Input: part model. Units: mm. Frame: model coordinates. Face numbers are marked on the shaded views. A direction names the side the tool comes from. Coordinates: 2 decimals unless noted, no trailing zeros. Write each loop counter-clockwise with the first axis right and the second up, starting at its lowest first coordinate (ties: lowest second). Pieces come first, ordered by that corner, then holes.
1) Pin query (flat end, axial travel): pin 1 Ø4.5 at (y, z) = (-0.5, 18.5) entering from +X. Return the tip coordinate at first contact, or that it passes through.
2) Section query B-B (y = 0). Output: boundary loops of the cut face in (x, z), then the cut area to 3 significant figures.
3) Section query A-A (x = 11). Output: boundary loops of the cut face in (y, z).
4) Draft query along X for the marked faces 1, 2, 3 and 4. Return one class per face: pulls with the +X half, pulls with the -X half, needs draft (parallel to the pull), parting line crosses it, or undercut.
5) Set-up query: the marked faces 5, 6 and 7. Return all of +Z, -Z, +X, -X, +Y, -Y with unobstructed straight access to the full face (end or side cutting, diameter ignored); none if empty.
6) Line query: L1, parallel to Y at x = -0.5, z = 6.5; L2, parallel to X at y = 2, z = 4.75; L3, parallel to Y at x = 18, z = 14. Output: solid intervals per line, ascending.
7) Section query D-D (z = 8.5). Output: boundary loops of the cut face in (x, y).
8) Section query C-C (z = 18.75). Output: boundary loops of the cut face in (x, y).
from build123d import *

# Parameters (mm, degrees)
F0_W     = 46
F0_H     = 35
F1_DEPTH = 30
F3_DEPTH = 6.251
F4_R     = 5


with BuildPart() as f1:
    # F0 (on Top) → F1 (new body)
    with BuildSketch(Plane.XY):
        Rectangle(F0_W, F0_H)
        Polygon((-17, 7.5), (-13, 11.5), (13, 11.5), (17, 7.5), (17, -7.5), (13, -11.5), (-13, -11.5), (-17, -7.5), align=None, mode=Mode.SUBTRACT)
    extrude(amount=F1_DEPTH)

    # F2 (on face) → F3 (cut, through all)
    with BuildSketch(Plane.YZ.offset(23)):
        with BuildLine():
            Line((-7.75, 30), (-7.75, 13.75))
            ThreePointArc((-7.75, 13.75), (0, 6), (7.75, 13.75))
            Line((7.75, 13.75), (7.75, 30))
            Line((7.75, 30), (-7.75, 30))
        make_face()
    extrude(amount=-F3_DEPTH, mode=Mode.SUBTRACT)

    # F4
    f4_edges = [f1.edges().sort_by_distance(p)[0] for p in [
        (23, -17.5, 15),
        (23, 17.5, 15),
        (-23, 17.5, 15),
        (-23, -17.5, 15),
    ]]
    fillet(f4_edges, radius=F4_R)


solid = f1.part
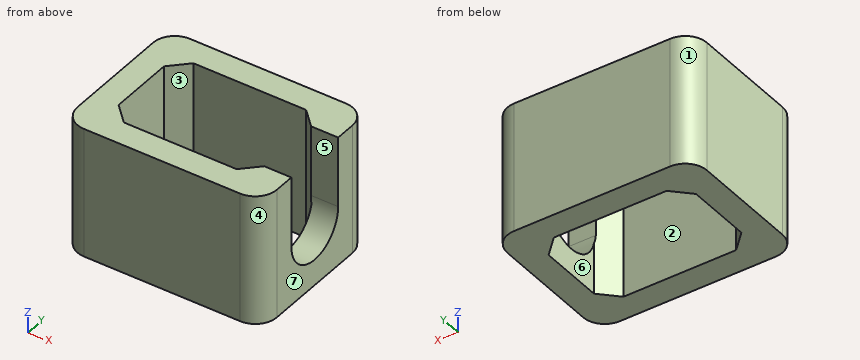
Answer:
1. pin 1: stops at x = -17
2. outline: (-23, 0) - (-17, 0) - (-17, 30) - (-23, 30) - close; (17, 0) - (23, 0) - (23, 6) - (17, 6) - close
2. area: 216 mm2
3. outline: (-17.5, 0) - (-11.5, 0) - (-11.5, 30) - (-17.5, 30) - close; (11.5, 0) - (17.5, 0) - (17.5, 30) - (11.5, 30) - close
4. face 1: pulls with the -X half
4. face 2: undercut
4. face 3: undercut
4. face 4: pulls with the +X half
5. face 5: +Z, +X
5. face 6: +Z, -Z
5. face 7: +Z, -Z, +X, +Y, -Y
6. L1: y = -17.5 to -11.5, 11.5 to 17.5
6. L2: x = -23 to -17, 17 to 23
6. L3: y = -17.5 to -7.75, 7.75 to 17.5
7. outline: (-23, -12.5) arc R5 ccw to (-18, -17.5) - (18, -17.5) arc R5 ccw to (23, -12.5) - (23, -5.7) - (17, -5.7) - (17, -7.5) - (13, -11.5) - (-13, -11.5) - (-17, -7.5) - (-17, 7.5) - (-13, 11.5) - (13, 11.5) - (17, 7.5) - (17, 5.7) - (23, 5.7) - (23, 12.5) arc R5 ccw to (18, 17.5) - (-18, 17.5) arc R5 ccw to (-23, 12.5) - close
8. outline: (-23, -12.5) arc R5 ccw to (-18, -17.5) - (18, -17.5) arc R5 ccw to (23, -12.5) - (23, -7.75) - (16.75, -7.75) - (13, -11.5) - (-13, -11.5) - (-17, -7.5) - (-17, 7.5) - (-13, 11.5) - (13, 11.5) - (16.75, 7.75) - (23, 7.75) - (23, 12.5) arc R5 ccw to (18, 17.5) - (-18, 17.5) arc R5 ccw to (-23, 12.5) - close
